Design review of the part built by this model. Coordinates are the model's own, in mm. A direction names the side the tool comes from. Give positions to 0.01 mm unless a question says otherwise; leave off trailing zeros. Write each loop counter-clockwise with the first axis right and the second up, starting at its lowest first coordinate (ties: lowest second). Pieces come first, ordered by that corner, then holes.
Autodesk Inventor part; units mm, degrees
ref_plane "YZ Plane" through (0, 0, 0) normal (1, 0, 0) x (0, 1, 0)
ref_plane "XZ Plane" through (0, 0, 0) normal (0, 1, 0) x (-1, 0, 0)
ref_plane "XY Plane" through (0, 0, 0) normal (0, 0, 1) x (1, 0, 0)
sketch "Sketch2" plane through (0, 0, 0) normal (0, 1, 0) x (-1, 0, 0)
  line L0 (12.7, 12.7) -> (-12.7, 12.7)
  line L1 (-12.7, 12.7) -> (-12.7, -12.7)
  line L2 (-12.7, -12.7) -> (12.7, -12.7)
  line L3 (12.7, -12.7) -> (12.7, 12.7)
  line L4 (12.7, 0) -> (-12.7, 0) construction
  line L5 (0, -12.7) -> (0, 12.7) construction
  point P0 (0, 0)
  point P1 (0, 0)
  dimension "d2" = 25.4
  dimension "d3" = 25.4
extrude "Base" add sketch "Sketch2" against normal blind 6.5
sketch "Sketch3" plane through (0, -6.5, 0) normal (0, -1, 0) x (1, 0, 0)
  line L0 (12.7, 12.7) -> (-12.7, 12.7)
  line L1 (12.7, 12.7) -> (6.35, 12.7)
  line L2 (6.35, 12.7) -> (6.35, 0)
  line L3 (6.35, 0) -> (12.7, 0)
  line L4 (12.7, 0) -> (12.7, 12.7)
  line L5 (0, 12.7) -> (6.35, 12.7)
  line L6 (6.35, 12.7) -> (6.35, 6.35)
  line L7 (6.35, 6.35) -> (0, 6.35)
  line L8 (0, 6.35) -> (0, 12.7)
  line L9 (-12.7, 12.7) -> (-12.7, -12.7)
  line L10 (12.7, 12.7) -> (-12.7, 12.7)
  line L11 (-12.7, 12.7) -> (-12.7, -12.7)
  line L12 (-12.7, -12.7) -> (12.7, -12.7)
  line L13 (12.7, -12.7) -> (12.7, 12.7)
  point P0 (0, 0)
  dimension "d6" = 6.35
  dimension "d7" = 12.7
extrude "Back extrusion" add sketch "Sketch3" along normal blind 6.5 contours L4 L3 L2 L0 | L2 L7 L8 L0
sketch "Sketch5" plane through (-12.7, 0, 12.7) normal (0, 0, 1) x (1, 0, 0)
  line L0 (12.7, -6.5) -> (0, -6.5)
  line L1 (25.4, -6.5) -> (25.4, -13)
  line L2 (12.7, -6.5) -> (25.4, -6.5) construction
  line L3 (25.4, -13) -> (12.7, -13)
  line L4 (25.4, -13) -> (20.4, -13) construction
  line L5 (20.4, -13) -> (20.4, -8) construction
  line L6 (20.4, -8) -> (25.4, -8) construction
  line L7 (25.4, -8) -> (25.4, -13) construction
  line L8 (20.4, -8) -> (25.4, -13) construction
  line L9 (20.4, -13) -> (25.4, -8) construction
  circle A0 centre (22.9, -10.5) radius 2.425
  point P0 (12.7, 0)
  dimension "d10" = 5
  dimension "d11" = 5
  dimension "d12" = 4.85
extrude "Extrusion3" add sketch "Sketch5" along normal blind 6.75
sketch "Sketch6" plane through (0, -6.5, 0) normal (0, -1, 0) x (1, 0, 0)
  line L0 (-12.7, 12.7) -> (-12.7, -12.7)
  line L1 (-12.7, -12.7) -> (-4.9218, -4.9218) construction
  line L2 (-12.7, -12.7) -> (-1.7, -12.7) construction
  line L3 (-4.9218, -4.9218) -> (-3.1541, -3.1541) construction
  line L4 (-4.9218, -4.9218) -> (-2.4218, -4.9218) construction
  circle A0 centre (-3.1541, -3.1541) radius 2.5
  point P0 (0, 0)
  dimension "d15" = 11
  dimension "d16" = 45
  dimension "d17" = 2.5
  dimension "d18" = 45
sketch "Sketch7" plane through (0, 0, 0) normal (0, 1, 0) x (1, 0, 0)
  line L0 (-12.7, -12.7) -> (-12.7, 12.7)
  line L1 (-12.7, 12.7) -> (-7.0431, 7.0431) construction
  line L2 (-12.7, 12.7) -> (-4.7, 12.7) construction
  line L3 (-7.0431, 7.0431) -> (-3.1541, 3.1541) construction
  line L4 (-7.0431, 7.0431) -> (-1.5431, 7.0431) construction
  circle A0 centre (-3.1541, 3.1541) radius 5.5
  point P0 (0, 0)
  dimension "d19" = 8
  dimension "d20" = 45
  dimension "d21" = 5.5
  dimension "d22" = 45
hole "Hole1" at (-3.1541, 0, -3.1541) direction (0, -1, 0) diameter 5.5 end through all countersink diameter 11 countersink angle 90
equation "\"d3\" = d2"
equation "\"d7\" = 2 * d6"
equation "\"d11\" = d10"
properties part number "Door pin right"
(1) Tool access review of faces 4 (the face through (12.7, -5, 3)), 5 (the face through (9, -10, 0)), 6 (the face through (9.884, -12.904, 16.028)), 7 (the face through (3, -10, 6.35)), 8 (the face through (-0.47, -4.65, -3.75)): name each direction out of +Z, -Z, +X, -X, +Y, -Y from which nothing blocks a thin tool from reaching the whole face with its end or side.
Resolved:
face 4: +Z, -Z, +X, +Y, -Y
face 5: -Z, +X, -X, -Y
face 6: +Z
face 7: -Z, -X, -Y
face 8: +Y, -Y
(2) Clearance check with flat-ended pins moving along their axes: P1, Ø3, axis at x = 4.5, y = -9.5, coming from the -Z side; P2, Ø3, axis at x = 9, y = -4.5, coming from the +Z side; P3, Ø4, axis at x = -6, z = -9.5, coming from the -Y side; P4, Ø7, axis at y = -9, z = 4.5, coming from the -X side. State where each tip first meets the part, or that it passes through.
Resolved:
P1: stops at z = 6.35
P2: stops at z = 12.7
P3: stops at y = -6.5
P4: stops at x = -12.7
(3) Consider section C-C, the plane y = -10.5. Give the boundary of the cut face in (x, z) (3 decimals), then the cut area to 3 significant figures.
Resolved:
outline: (0, 6.35) - (6.35, 6.35) - (6.35, 0) - (12.7, 0) - (12.7, 12.7) - (12.625, 12.7) - (12.625, 19.45) - (7.775, 19.45) - (7.775, 12.7) - (0, 12.7) - close
area: 154 mm2
(4) Consider section A-A, the plane x = 10.2. Give the boundary of the cut face in (y, z) (3 decimals).
Resolved:
outline: (-13, 0) - (-6.5, 0) - (-6.5, -12.7) - (0, -12.7) - (0, 12.7) - (-8.075, 12.7) - (-8.075, 19.45) - (-12.925, 19.45) - (-12.925, 12.7) - (-13, 12.7) - close
(5) To check wall thickness, follow L1, parallel to Y at x = -10.5, z = -5; L2, parallel to Z at x = 3, y = -2.25; L3, parallel to Z at x = 0.25, y = -10. State the ranges of each line that lie inside material, in increasing order.
Resolved:
L1: y = -6.5 to 0
L2: z = -12.7 to 12.7
L3: z = 6.35 to 12.7
(6) Consider section B-B, the plane z = 12. Give the boundary of the cut face in (x, y), then the cut area to 3 significant figures.
Resolved:
outline: (-12.7, -6.5) - (0, -6.5) - (0, -13) - (12.7, -13) - (12.7, 0) - (-12.7, 0) - close
area: 248 mm2
(7) Mouldability with a two-part tool opening along X and no side actions: class faces 1 (the face through (-2.28, -2.58, -0.37)), 2 (the face through (0, 0, 3)), 3 (the face through (0, -10, 9)) as pulls with the +X half, pulls with the -X half, needs draft (parallel to the pull), parting line crosses it, or undercut.
Resolved:
face 1: undercut
face 2: needs draft
face 3: pulls with the -X half
(8) Consider section D-D, the plane z = 3. Give the boundary of the cut face in (x, y), then the cut area to 3 significant figures.
Resolved:
outline: (-12.7, -6.5) - (6.35, -6.5) - (6.35, -13) - (12.7, -13) - (12.7, 0) - (-12.7, 0) - close
area: 206 mm2
